CAD build for the part. Positions are in the model's coordinates, mm. A direction names the side the tool comes from. Give positions to 0.01 mm unless a question says otherwise; leave off trailing zeros. Write each loop counter-clockwise with the first axis right and the second up, starting at its lowest first coordinate (ties: lowest second). Pieces come first, ordered by that corner, then holes. Notation, with made-up numbers: (55.25, 77.25) - (114.25, 77.25) arc R35 ccw to (114.25, 110.25) - close; hole circle Ø2 at (15.25, -20). An arc over 180 degrees is marked (long way). Put each result on its own line as item: value. Start each with the question number.
1. Mould opens along Y. For faces 4 (the flat face through (0, 0, 3.8)), 5 (the cylindrical face through (-1.08, -4.88, 2.03)), 6 (the cylindrical face through (-3.746, 0.165, 1.479)) say: +Y half, -Y half, draft (parallel to the pull), parting line (faces both ways), or undercut.
2. Tool access for faces 1 (the cylindrical face through (-0.1, -6, 0.4)), 2 (the flat face through (-4, -4, 0.8)), 3 (the flat face through (0, 0, 3)): list every direction of +Z, -Z, +X, -X, +Y, -Y with a clear straight run to the whole face (end or side of a thin tool).
3. Cut at C-C on y = 0. List the corners of the cut face in (x, z), and give its area (3 significant figures).
4. Drop flat-ended pins along their axis: pin 1 (2 mm diameter, centred on x = 1, z = 1.5, fed in from -Y); pin 2 (4 mm diameter, centred on x = -1.5, y = -0.5, fed in from -Z); pin 3 (1.5 mm diameter, centred on y = -2.5, z = 2.5, fed in from +X). Give the stop position or say it passes through.
5. Wall check: line 1 (Y direction, x = 0, z = 1.1); line 2 (Z direction, x = 1, y = 3.5); line 3 (Y direction, x = -2.75, z = 0.75). Give the ranges that are in metal, low to high.
6. Cut at B-B on x = 0. List the corners of the cut face in (y, z), and give its area (3 significant figures).
7. Cut at A-A on z = 1.7. List the corners of the cut face in (x, y).
from build123d import *

# Parameters (mm, degrees)
SKETCH_2_R      = 5
EXTRUDE_1_DEPTH = 0.8
SKETCH_2_3_R    = 5
SKETCH_2_3_R_2  = 3.75
EXTRUDE_2_DEPTH = 3.8
SKETCH_3_R      = 3.75
EXTRUDE_3_DEPTH = 0.8
FILLET_1_R      = 0.5


with BuildPart() as part:
    # Sketch 2 → Extrude 1 (new body)
    with BuildSketch(Plane.XY):
        with BuildLine():
            Line((-5.4, 2.615339366), (-5.4, -2.615339366))
            ThreePointArc((-5.4, -2.615339366), (0, -6), (5.4, -2.615339366))
            Line((5.4, -2.615339366), (5.4, 2.615339366))
            ThreePointArc((5.4, 2.615339366), (0, 6), (-5.4, 2.615339366))
        make_face()
        Circle(SKETCH_2_R, mode=Mode.SUBTRACT)
    extrude(amount=EXTRUDE_1_DEPTH)

    # Sketch 2_3 → Extrude 2 (add)
    with BuildSketch(Plane.XY):
        Circle(SKETCH_2_3_R)
        Circle(SKETCH_2_3_R_2, mode=Mode.SUBTRACT)
    extrude(amount=EXTRUDE_2_DEPTH)

    # Sketch 3 → Extrude 3 (add)
    with BuildSketch(Plane.XY.offset(3.8)):
        Circle(SKETCH_3_R)
    extrude(amount=-EXTRUDE_3_DEPTH)

    # Fillet 1
    fillet_1_edges = [part.edges().sort_by_distance(p)[0] for p in [
        (-5, 0, 3.8),
    ]]
    fillet(fillet_1_edges, radius=FILLET_1_R)


solid = part.part
Report:
1. face 4: draft
1. face 5: parting line
1. face 6: undercut
2. face 1: +Z, -Z, -Y
2. face 2: +Z
2. face 3: -Z
3. outline: (-5.4, 0) - (-3.75, 0) - (-3.75, 3) - (3.75, 3) - (3.75, 0) - (5.4, 0) - (5.4, 0.8) - (5, 0.8) - (5, 3.3) arc R0.5 ccw to (4.5, 3.8) - (-4.5, 3.8) arc R0.5 ccw to (-5, 3.3) - (-5, 0.8) - (-5.4, 0.8) - close
3. area: 16.0 mm²
4. pin 1: stops at y = -5.99
4. pin 2: stops at z = 3
4. pin 3: stops at x = 4.68
5. line 1: y = -5 to -3.75, 3.75 to 5
5. line 2: z = 3 to 3.8
5. line 3: y = -5.33 to -2.55, 2.55 to 5.33
6. outline: (-6, 0) - (-3.75, 0) - (-3.75, 3) - (3.75, 3) - (3.75, 0) - (6, 0) - (6, 0.8) - (5, 0.8) - (5, 3.3) arc R0.5 ccw to (4.5, 3.8) - (-4.5, 3.8) arc R0.5 ccw to (-5, 3.3) - (-5, 0.8) - (-6, 0.8) - close
6. area: 17.0 mm²
7. outline: circle Ø10 at (0, 0); hole circle Ø7.5 at (0, 0)
